from build123d import *

# Parameters (mm, degrees)
SKETCH1_W           = 30
SKETCH1_H           = 25
SKETCH1_W_2         = 7
SKETCH1_H_2         = 3
BOSS_EXTRUDE1_DEPTH = 3
CUT_EXTRUDE1_DEPTH  = 4
FILLET1_R           = 1


with BuildPart() as part:
    # Sketch1 → Boss-Extrude1 (new body)
    with BuildSketch(Plane(origin=(0, 0, 0), x_dir=(1, 0, 0), z_dir=(0, 1, 0))):
        Rectangle(SKETCH1_W, SKETCH1_H)
        with Locations((-7, -14)):
            Rectangle(SKETCH1_W_2, SKETCH1_H_2)
        with Locations((7, -14)):
            Rectangle(SKETCH1_W_2, SKETCH1_H_2)
    extrude(amount=BOSS_EXTRUDE1_DEPTH)

    # Sketch2 → Cut-Extrude1 (cut, through all)
    with BuildSketch(Plane(origin=(0, 3, 0), x_dir=(1, 0, 0), z_dir=(0, 1, 0))):
        with BuildLine():
            Line((-4.472135955, 12.5), (-15, 12.5))
            Line((-15, 12.5), (-15, -2.54996447))
            add(Edge.make_bspline(
                [(-15, -2.54996447), (-11.338987125, 2.558357454), (-12.102816027, 10.660548238), (-4.472135955, 12.5)],
                knots=[0, 0, 0, 0, 1, 1, 1, 1], degree=3))
        make_face()
        with BuildLine():
            Line((6, 8.5), (6, -2.5))
            ThreePointArc((6, -2.5), (0, -8.5), (-6, -2.5))
            Line((-6, -2.5), (-6, 8.5))
            ThreePointArc((-6, 8.5), (0, 14.5), (6, 8.5))
        make_face()
        with BuildLine():
            Line((15, 12.5), (15, -2.54996447))
            add(Edge.make_bspline(
                [(15, -2.54996447), (11.338987125, 2.558357454), (12.102816027, 10.660548238), (4.472135955, 12.5)],
                knots=[0, 0, 0, 0, 1, 1, 1, 1], degree=3))
            Line((4.472135955, 12.5), (15, 12.5))
        make_face()
    extrude(amount=-CUT_EXTRUDE1_DEPTH, mode=Mode.SUBTRACT)

    # Fillet1
    fillet1_edges = [part.edges().sort_by_distance(p)[0] for p in [
        (-4.472135955, 1.5, -12.5),
        (4.472135955, 1.5, -12.5),
    ]]
    fillet(fillet1_edges, radius=FILLET1_R)


solid = part.part
Here's how the part is built. I have some questions about the finished solid (model axes, mm). A direction names the side the tool comes from. Give positions to 0.01 mm unless a question says otherwise; leave off trailing zeros. Order: outer loops, then holes, each group sorted by start corner. A loop starts at its lowest first (then second) coordinate and runs counter-clockwise, first axis right, second up. Notation, with made-up numbers: (43, -35) -> (97, -35) arc R20 ccw to (97, -30) -> close; hole circle Ø4 at (44, 8). An arc over 180 degrees is marked (long way). Use a Markdown table: item, result. Add a question column.
Item 1: If we mould it in two halves opening along Z, with no side actions, what happens to faces 1 (the face through (-4, 3, 8)), 2 (the face through (13, 1, 12.5)), 3 (the face through (6, 2, -3))? For each: pulls with the +Z half, pulls with the -Z half, needs draft (parallel to the pull), parting line crosses it, or undercut.
Item 2: For faces 4 (the face through (10.5, 1, 14)), 5 (the face through (-4, 0, 8)), 6 (the face through (0, 1, 12.5)), 7 (the face through (0.1, 1.5, 8.5)), 8 (the face through (-13, 1, 12.5)), which set-ups out of +Z, -Z, +X, -X, +Y, -Y let a thin tool reach every point of the face, with its end or its side?
Item 3: I need wall thicknesses on line 1 (X direction, y = 1.9, z = 14.5); line 2 (X direction, y = 1.95, z = -5.75); line 3 (Z direction, x = 1, y = 1.9). Which ranges of each line are inside material? Lowest first, please.
Item 4: Imagine slicing it at B-B on x = -5. Please give me the cut outline in (y, z), plus the area to 3 significant figures.
Item 5: Imagine slicing it at A-A on x = 0. Please give me the cut outline in (y, z), plus the area to 3 significant figures.
Item 6: Will these pins go through, and if not, where does the flat tip stop? pin 1 (0.9 mm diameter, centred on y = 1, z = -5.5, fed in from -X); pin 2 (0.9 mm diameter, centred on x = -13, y = 1, fed in from +Z); pin 3 (3 mm diameter, centred on x = 2.5, z = 3, fed in from +Y); pin 4 (1 mm diameter, centred on y = 1, z = -1.5, fed in from +X).
Data:
| question | item | result |
|---|---|---|
| 1 | face 1 | needs draft |
| 1 | face 2 | pulls with the +Z half |
| 1 | face 3 | undercut |
| 2 | face 4 | +Z, +X, +Y, -Y |
| 2 | face 5 | +Z, -Z, +X, -X, -Y |
| 2 | face 6 | +Z, +Y, -Y |
| 2 | face 7 | +Y, -Y |
| 2 | face 8 | +Z, -X, +Y, -Y |
| 3 | line 1 | x = -10.5 to -3.5, 3.5 to 10.5 |
| 3 | line 2 | x = -11.41 to -6, 6 to 11.41 |
| 3 | line 3 | z = 8.42 to 12.5 |
| 4 | outline | (0, 5.82) -> (3, 5.82) -> (3, 15.5) -> (0, 15.5) -> close |
| 4 | area | 29.1 mm² |
| 5 | outline | (0, 8.5) -> (3, 8.5) -> (3, 12.5) -> (0, 12.5) -> close |
| 5 | area | 12.0 mm² |
| 6 | pin 1 | stops at x = -11.68 |
| 6 | pin 2 | stops at z = 12.5 |
| 6 | pin 3 | passes through |
| 6 | pin 4 | stops at x = 13.15 |
